Check sheet for the modelled part. Datum: model origin and axes. Units: mm. A direction names the side the tool comes from. Coordinates: 2 decimals unless noted, no trailing zeros. Write each loop counter-clockwise with the first axis right and the second up, starting at its lowest first coordinate (ties: lowest second). Pieces come first, ordered by that corner, then holes. Notation, with made-up numbers: M 6,55.5 L 14,55.5 A34 ccw 14,91.5 Z; hole C -24,-21.75 d2. An arc over 180 degrees is marked long. Answer as CSV lines item,"result". Start each with the question number.
Q1. Mould release check, pull along Z, two halves, no side actions. Record for faces 3 (the flat face through (1, 0, -110)), 4 (the cylindrical face through (23.846, 7.509, 499.16)), 5 (the flat face through (5.2, -5.2, 440)): pulls with the +Z half, pulls with the -Z half, needs draft (parallel to the pull), parting line crosses it, or undercut.
Q2. Sectioned sample at B-B, the plane x = 70. Record the cut outline in (y, z) (3 decimals), then the cut area to 3 significant figures.
Q3. Access from +Z, -Z, +X, -X, +Y, -Y to the whole of each face (thin tool, end or side, straight path). Record for faces 1 (the flat face through (143.318, 0, -100)), 2 (the cylindrical face through (-113.077, 3.755, -381.245)).
Q4. Thickness scan on line 1 along Z through (x, y) = (-15, 9.5); line 2 along Y through (x, z) = (-51, -108.5) (3 decimals); line 3 along Z through (x, y) = (-26.5, -13). Record the ranges inside material, lowest first. Write a range as from..to.
Q5. Depth check by flat-ended pin: pin 1 Ø21 at (x, y) = (-63.5, 5) entering from +Z; pin 2 Ø4 at (y, z) = (-7, -18.5) entering from -X; pin 3 Ø8 at (y, z) = (3.5, 352) entering from -X. Enter the tip coordinate at first touch or a pass-through.
Q6. Sectioned sample at C-C, the plane z = 104. Record the cut outline in (x, y), then the cut area to 3 significant figures.
Q7. Sectioned sample at A-A, the plane z = -299. Record the cut outline in (x, y).
from build123d import *

# Parameters (mm, degrees)
BOSS_EXTRUDE1_DEPTH      = 500
BOSS_EXTRUDE1_DEPTH_BACK = 100
SKETCH1_R                = 7
SKETCH4_R                = 12.5
BOSS_EXTRUDE2_DEPTH      = 550
BOSS_EXTRUDE2_2_DEPTH    = 550
BOSS_EXTRUDE3_DEPTH      = 10
BOSS_EXTRUDE3_DEPTH_BACK = 10
SKETCH5_W                = 288.220289941
SKETCH5_H                = 26.942823647
FILLET4_R                = 0.5
FILLET8_R                = 0.5
FILLET9_R                = 5
BOSS_EXTRUDE4_DEPTH      = 60
BOSS_EXTRUDE4_DEPTH_BACK = 60
SKETCH6_R                = 25


with BuildPart() as part:
    # Sketch1 → Boss-Extrude1 (new, two sides: drawn at the far end of the back side and taken through both)
    with BuildSketch(Plane.XY.offset(-BOSS_EXTRUDE1_DEPTH_BACK)):
        Circle(SKETCH1_R)
    extrude(amount=BOSS_EXTRUDE1_DEPTH + BOSS_EXTRUDE1_DEPTH_BACK)



with BuildPart() as body_2:
    # Sketch4 → Boss-Extrude2 (new body)
    with BuildSketch(Plane.XY.offset(-650)):
        with Locations((-125, 0)):
            Circle(SKETCH4_R)
    extrude(amount=BOSS_EXTRUDE2_DEPTH)


with BuildPart() as body_3:
    # Sketch4 → Boss-Extrude2 2 (new body)
    with BuildSketch(Plane.XY.offset(-650)):
        with Locations((125, 0)):
            Circle(SKETCH4_R)
    extrude(amount=BOSS_EXTRUDE2_2_DEPTH)


with BuildPart() as part_1:
    add(part.part)

    add(body_2.part)  # Boss-Extrude3 merges body 2

    add(body_3.part)  # Boss-Extrude3 merges body 3
    # Sketch5 → Boss-Extrude3 (add, two sides: drawn at the far end of the back side and taken through both)
    with BuildSketch(Plane(origin=(0, 0, -100), x_dir=(-1, 0, 0), z_dir=(0, 0, -1)).offset(-BOSS_EXTRUDE3_DEPTH_BACK)):
        with Locations((0.79243599, -0.226410282)):
            Rectangle(SKETCH5_W, SKETCH5_H)
    extrude(amount=BOSS_EXTRUDE3_DEPTH + BOSS_EXTRUDE3_DEPTH_BACK)

    # Fillet4
    fillet4_edges = [part_1.edges().sort_by_distance(p)[0] for p in [
        (-7, 0, -90),
    ]]
    fillet(fillet4_edges, radius=FILLET4_R)

    # Fillet8
    fillet8_edges = [part_1.edges().sort_by_distance(p)[0] for p in [
        (-144.90258096, 13.245001541, -100),
        (-144.90258096, -0.226410283, -90),
        (-144.90258096, -13.697822106, -100),
        (-0.79243599, -13.697822106, -90),
        (143.317708981, -0.226410283, -110),
        (-0.79243599, -13.697822106, -110),
        (-144.90258096, -0.226410283, -110),
        (-0.79243599, 13.245001541, -110),
        (143.317708981, -13.697822106, -100),
        (143.317708981, -0.226410283, -90),
        (143.317708981, 13.245001541, -100),
        (-0.79243599, 13.245001541, -90),
    ]]
    fillet(fillet8_edges, radius=FILLET8_R)

    # Fillet9
    fillet9_edges = [part_1.edges().sort_by_distance(p)[0] for p in [
        (-137.5, 0, -650),
        (112.5, 0, -650),
    ]]
    fillet(fillet9_edges, radius=FILLET9_R)

    # Sketch6 → Boss-Extrude4 (add, two sides: drawn at the far end of the back side and taken through both)
    with BuildSketch(Plane.XY.offset(500).offset(-BOSS_EXTRUDE4_DEPTH_BACK)):
        Circle(SKETCH6_R)
    extrude(amount=BOSS_EXTRUDE4_DEPTH + BOSS_EXTRUDE4_DEPTH_BACK)


solid = part_1.part
Output:
1,face 3,"pulls with the -Z half"
1,face 4,"needs draft"
1,face 5,"undercut"
2,outline,"M -13.698,-109.5 A0.5 ccw -13.198,-110 L 12.745,-110 A0.5 ccw 13.245,-109.5 L 13.245,-90.5 A0.5 ccw 12.745,-90 L -13.198,-90 A0.5 ccw -13.698,-90.5 Z"
2,area,"539 mm^2"
3,face 1,"+Z, -Z, +X, +Y, -Y"
3,face 2,"-Z"
4,line 1,"z = -110..-90, 440..560"
4,line 2,"y = -13.698..13.245"
4,line 3,"z = -110..-90"
5,pin 1,"stops at z = -90"
5,pin 2,"stops at x = -4.9"
5,pin 3,"stops at x = -7"
6,outline,"C 0,0 d14"
6,area,"154 mm^2"
7,outline,"C -125,0 d25; C 125,0 d25"
